```python
from build123d import *

# Parameters (mm, degrees)
F0_R     = 225
F1_DEPTH = 2
F3_D     = 6.5
F5_DEPTH = 2.001


# Not quite as in the source:
# - a feature names something its author has since deleted; it is built from what else it names


with BuildPart() as f1:
    # F0 (on Top) → F1 (new body)
    with BuildSketch(Plane.XY):
        Circle(F0_R)
    extrude(amount=F1_DEPTH)

    # F3 (through all)
    with Locations(Plane.XY.offset(2)):
        with Locations((219, 0), (205.7926839521, 74.9024113883), (167.7637330431, 140.7704865214), (109.5, 189.6595634288), (38.0289509091, 215.6728979097), (-38.0289509091, 215.6728979097), (-109.5, 189.6595634288), (-167.7637330431, 140.7704865214), (-205.7926839521, 74.9024113883), (-219, 0), (-205.7926839521, -74.9024113883), (-167.7637330431, -140.7704865214), (-109.5, -189.6595634288), (-38.0289509091, -215.6728979097), (38.0289509091, -215.6728979097), (109.5, -189.6595634288), (167.7637330431, -140.7704865214), (205.7926839521, -74.9024113883)):
            Hole(F3_D / 2)

    # F4 (on face) → F5 (cut, through all)
    with BuildSketch(Plane.XY.offset(2)):
        with BuildLine():
            ThreePointArc((223.6935148816, 24.2118029049), (221.5817444277, 39.0708399751), (218.4840695516, 53.7560354952))
            Line((218.4840695516, 53.7560354952), (208.6359920215, 52.0195537186))
            ThreePointArc((208.6359920215, 52.0195537186), (207.3449842883, 51.1970910852), (207.0136728708, 49.7026418572))
            Line((207.0136728708, 49.7026418572), (209.2710991805, 36.900141068))
            Line((209.2710991805, 36.900141068), (211.5285254901, 24.0976402789))
            ThreePointArc((211.5285254901, 24.0976402789), (212.3509881235, 22.8066325456), (213.8454373515, 22.4753211282))
            Line((213.8454373515, 22.4753211282), (223.6935148816, 24.2118029049))
        make_face()
        with BuildLine():
            Line((149.3682510245, 154.6742923751), (155.7961271214, 162.3347368063))
            ThreePointArc((155.7961271214, 162.3347368063), (144.6272121795, 172.3599997018), (132.8147938278, 181.6183650969))
            Line((132.8147938278, 181.6183650969), (126.386917731, 173.9579206657))
            ThreePointArc((126.386917731, 173.9579206657), (125.926617221, 172.4980339608), (126.6334313978, 171.1402565601))
            Line((126.6334313978, 171.1402565601), (136.5920091584, 162.7840176342))
            Line((136.5920091584, 162.7840176342), (146.5505869189, 154.4277787082))
            ThreePointArc((146.5505869189, 154.4277787082), (148.0104736238, 153.9674781983), (149.3682510245, 154.6742923751))
        make_face()
        with BuildLine():
            Line((15, 214.4994432064), (15, 224.4994432064))
            ThreePointArc((15, 224.4994432064), (0, 225), (-15, 224.4994432064))
            Line((-15, 224.4994432064), (-15, 214.4994432064))
            ThreePointArc((-15, 214.4994432064), (-14.4142135624, 213.0852296441), (-13, 212.4994432064))
            Line((-13, 212.4994432064), (0, 212.4994432064))
            Line((0, 212.4994432064), (13, 212.4994432064))
            ThreePointArc((13, 212.4994432064), (14.4142135624, 213.0852296441), (15, 214.4994432064))
        make_face()
        with BuildLine():
            Line((-126.386917731, 173.9579206657), (-132.8147938278, 181.6183650969))
            ThreePointArc((-132.8147938278, 181.6183650969), (-144.6272121795, 172.3599997018), (-155.7961271214, 162.3347368063))
            Line((-155.7961271214, 162.3347368063), (-149.3682510245, 154.6742923751))
            ThreePointArc((-149.3682510245, 154.6742923751), (-148.0104736238, 153.9674781983), (-146.5505869189, 154.4277787082))
            Line((-146.5505869189, 154.4277787082), (-136.5920091584, 162.7840176342))
            Line((-136.5920091584, 162.7840176342), (-126.6334313978, 171.1402565601))
            ThreePointArc((-126.6334313978, 171.1402565601), (-125.926617221, 172.4980339608), (-126.386917731, 173.9579206657))
        make_face()
        with BuildLine():
            Line((-208.6359920215, 52.0195537186), (-218.4840695516, 53.7560354952))
            ThreePointArc((-218.4840695516, 53.7560354952), (-221.5817444277, 39.0708399751), (-223.6935148816, 24.2118029049))
            Line((-223.6935148816, 24.2118029049), (-213.8454373515, 22.4753211282))
            ThreePointArc((-213.8454373515, 22.4753211282), (-212.3509881235, 22.8066325456), (-211.5285254901, 24.0976402789))
            Line((-211.5285254901, 24.0976402789), (-209.2710991805, 36.900141068))
            Line((-209.2710991805, 36.900141068), (-207.0136728708, 49.7026418572))
            ThreePointArc((-207.0136728708, 49.7026418572), (-207.3449842883, 51.1970910852), (-208.6359920215, 52.0195537186))
        make_face()
        with BuildLine():
            ThreePointArc((-201.9222209522, -99.2593405465), (-194.8557158515, -112.5), (-186.9222209522, -125.24010266))
            Line((-186.9222209522, -125.24010266), (-178.2619669144, -120.24010266))
            ThreePointArc((-178.2619669144, -120.24010266), (-177.3301152618, -119.0256899426), (-177.5299161068, -117.5080518524))
            Line((-177.5299161068, -117.5080518524), (-184.0299161068, -106.2497216032))
            Line((-184.0299161068, -106.2497216032), (-190.5299161068, -94.991391354))
            ThreePointArc((-190.5299161068, -94.991391354), (-191.7443288242, -94.0595397014), (-193.2619669144, -94.2593405465))
            Line((-193.2619669144, -94.2593405465), (-201.9222209522, -99.2593405465))
        make_face()
        with BuildLine():
            ThreePointArc((-90.8787210538, -205.8301680017), (-76.9545322483, -211.4308396768), (-62.6879424302, -216.0907723015))
            Line((-62.6879424302, -216.0907723015), (-59.267740997, -206.6938460937))
            ThreePointArc((-59.267740997, -206.6938460937), (-59.3345106645, -205.1645692835), (-60.4630859519, -204.1304205654))
            Line((-60.4630859519, -204.1304205654), (-72.6790900221, -199.6841587022))
            Line((-72.6790900221, -199.6841587022), (-84.8950940923, -195.237896839))
            ThreePointArc((-84.8950940923, -195.237896839), (-86.4243709024, -195.3046665065), (-87.4585196205, -196.4332417939))
            Line((-87.4585196205, -196.4332417939), (-90.8787210538, -205.8301680017))
        make_face()
        with BuildLine():
            ThreePointArc((62.6879424302, -216.0907723015), (76.9545322483, -211.4308396768), (90.8787210538, -205.8301680017))
            Line((90.8787210538, -205.8301680017), (87.4585196205, -196.4332417939))
            ThreePointArc((87.4585196205, -196.4332417939), (86.4243709024, -195.3046665065), (84.8950940923, -195.237896839))
            Line((84.8950940923, -195.237896839), (72.6790900221, -199.6841587022))
            Line((72.6790900221, -199.6841587022), (60.4630859519, -204.1304205654))
            ThreePointArc((60.4630859519, -204.1304205654), (59.3345106645, -205.1645692835), (59.267740997, -206.6938460937))
            Line((59.267740997, -206.6938460937), (62.6879424302, -216.0907723015))
        make_face()
        with BuildLine():
            ThreePointArc((186.9222209522, -125.24010266), (194.8557158515, -112.5), (201.9222209522, -99.2593405465))
            Line((201.9222209522, -99.2593405465), (193.2619669144, -94.2593405465))
            ThreePointArc((193.2619669144, -94.2593405465), (191.7443288242, -94.0595397014), (190.5299161068, -94.991391354))
            Line((190.5299161068, -94.991391354), (184.0299161068, -106.2497216032))
            Line((184.0299161068, -106.2497216032), (177.5299161068, -117.5080518524))
            ThreePointArc((177.5299161068, -117.5080518524), (177.3301152618, -119.0256899426), (178.2619669144, -120.24010266))
            Line((178.2619669144, -120.24010266), (186.9222209522, -125.24010266))
        make_face()
    extrude(amount=-F5_DEPTH, mode=Mode.SUBTRACT)


solid = f1.part
```
Could you check a few things on this model? Use its own coordinates, in mm. A direction names the side the tool comes from. Round coordinates to 2 decimals unless told otherwise and drop trailing zeros. Loops run counter-clockwise (first coordinate to the right, second up) from the corner with the lowest first, then second, coordinate; pieces in that order, holes last. Notation, with made-up numbers: (-7, -22.5) -> (27, -22.5) arc R30 cw to (27, 14.5) -> close; hole circle Ø10 at (6, 56.5). An arc over 180 degrees is marked (long way). Put each result on its own line as item: value.
Q1. Which directions (+Z, -Z, +X, -X, +Y, -Y) give clear straight access to the entire face, cutting with the end or side of a thin tool? Please do faces 1 (the flat face through (-183.939, -106.407, 1.014)), 2 (the cylindrical face through (221.426, -39.946, 0.986)).
Checks:
face 1: +Z, -Z
face 2: +Z, -Z, +X
Q2. Thinking about a two-plate mould opening in Y: for faces 3 (the flat face through (184.12, -106.09, 1.01)), 4 (the cylindrical face through (195.3, 111.73, 0.99)), 5 (the cylindrical face through (143.945, -172.93, 0.986)), which applies, pulls with the +Y half, pulls with the -Y half, needs draft (parallel to the pull), parting line crosses it, or undercut?
Checks:
face 3: undercut
face 4: pulls with the +Y half
face 5: pulls with the -Y half
Q3. For pin 1 Ø7.5 at (x, y) = (38.03, 215.67) entering from +Z; pin 2 Ø1 at (x, z) = (6, 1) entering from +Y; pin 3 Ø1 at (x, z) = (49, 2) entering from +Y, each with a flat end and sliding along its axis, tell me the tip position at first contact or that it passes through.
Checks:
pin 1: z = 2
pin 2: y = 212.5
pin 3: y = 219.71
Q4. Please list where these lines run through material, in increasing order: line 1 (Y direction, x = -109.5, z = 1.05); line 2 (Y direction, x = 36, z = 1.2); line 3 (X direction, y = -142.5, z = 1). Write a range as from..to.
Checks:
line 1: -196.56..-192.91, -186.41..186.41, 192.91..196.56
line 2: -222.1..-218.21, -213.13..213.13, 218.21..222.1
line 3: -174.12..-170.52, -165.01..165.01, 170.52..174.12
Q5. I want a section at B-B on y = 113.5. Write out the boundary of the cut face in (x, z), and give its area (3 significant figures).
Checks:
outline: (-194.27, 0) -> (194.27, 0) -> (194.27, 2) -> (-194.27, 2) -> close
area: 777 mm2
Q6. I want a section at A-A on z = 0.45. Give the number of separate pieces and of enclosed holes in the cut face, and give its area (3 significant figures).
Checks:
separate pieces: 1
enclosed holes: 18
area: 155,000 mm2
